Source: CAD feature listing. Evaluate the final solid. Frame: model axes, mm. Face numbers are marked on the shaded views. Round coordinates to 2 decimals unless told otherwise and drop trailing zeros. Write each loop counter-clockwise with the first axis right and the second up, starting at its lowest first coordinate (ties: lowest second). Pieces come first, ordered by that corner, then holes.
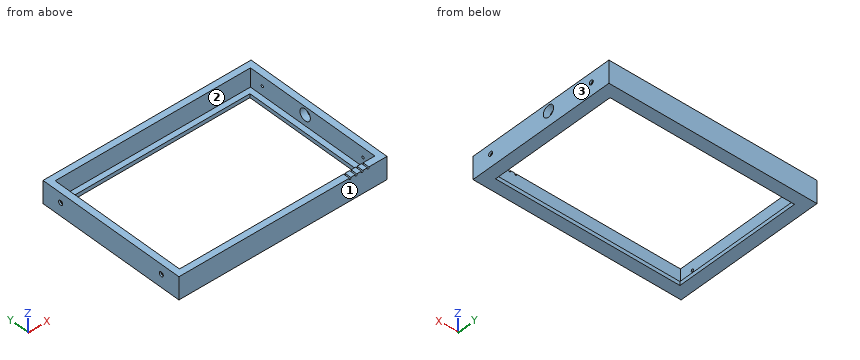
from build123d import *

# Parameters (mm, degrees)
CYLINDER027_R           = 3.5
CYLINDER027_DEPTH       = 3
CYLINDER027_PITCH_ANGLE = 90
CYLINDER026_R           = 2
CYLINDER026_DEPTH       = 9
CYLINDER026_PITCH_ANGLE = 90
ARRAY023_COUNT          = 2
ARRAY024_Y_COUNT        = 2
ARRAY024_Y_PITCH        = 174
CYLINDER011_R           = 9
CYLINDER011_DEPTH       = 12
CYLINDER011_PITCH_ANGLE = 90
CYLINDER010_R           = 1.5
CYLINDER010_DEPTH       = 11
ARRAY007_X_COUNT        = 4
ARRAY007_X_PITCH        = 9.4
ARRAY007_ROLL_ANGLE     = 90
BOX005_W                = 288
BOX005_H                = 198
BOX005_DEPTH            = 6
BOX004_W                = 325
BOX004_H                = 235
BOX004_DEPTH            = 6
BOX007_W                = 305
BOX007_H                = 215
BOX007_DEPTH            = 29
BOX006_W                = 325
BOX006_H                = 235
BOX006_DEPTH            = 29
CUT014_PLACEMENT_ANGLE  = 180


with BuildPart() as case_2_frame_cut005:
    # Cylinder027 → Cylinder027 (new body)
    with BuildSketch(Plane.XY):
        Circle(CYLINDER027_R)
    extrude(amount=CYLINDER027_DEPTH)


with BuildPart() as case_2_frame_cut005_1:
    # Cylinder027 pitch: moved
    add(case_2_frame_cut005.part.rotate(Axis((0, 0, 0), (0, 1, 0)), CYLINDER027_PITCH_ANGLE))


with BuildPart() as case_2_frame_cut005_2:
    # Cylinder027 placement: moved
    add(case_2_frame_cut005_1.part)


with BuildPart() as array024:
    # Cylinder026 → Cylinder026 (new body)
    with BuildSketch(Plane.XY):
        Circle(CYLINDER026_R)
    extrude(amount=CYLINDER026_DEPTH)


with BuildPart() as array024_1:
    # Cylinder026 pitch: moved
    add(array024.part.rotate(Axis((0, 0, 0), (0, 1, 0)), CYLINDER026_PITCH_ANGLE))


with BuildPart() as array024_2:
    # Cylinder026 placement: moved
    add(array024_1.part.moved(Location((3, 0, 0))))

    # Fusion021: union CASE_2_frame_cut005
    add(case_2_frame_cut005_2.part)


with BuildPart() as array024_3:
    # Fusion021 placement: moved
    add(array024_2.part.moved(Location((-163, 87, -14))))

    # Array023: Array024 ×2 about axis
    array023_axis = Axis((0, 87, 0), (0, 0, 1))


with BuildPart() as array024_4:
    add(array024_3.part)
    for i in range(1, ARRAY023_COUNT):
        add(array024_3.part.rotate(array023_axis, i * 360 / ARRAY023_COUNT))

    # Array024 Y: Array024 ×2


with BuildPart() as array024_5:
    add(array024_4.part)
    with Locations(*[(0, -i * ARRAY024_Y_PITCH, 0) for i in range(1, ARRAY024_Y_COUNT)]):
        add(array024_4.part)


with BuildPart() as array024_6:
    # Array024 placement: moved
    add(array024_5.part.moved(Location((0, 0, -30))))


with BuildPart() as case_2_frame_cut:
    # Cylinder011 → Cylinder011 (new body)
    with BuildSketch(Plane.XY):
        Circle(CYLINDER011_R)
    extrude(amount=CYLINDER011_DEPTH)


with BuildPart() as case_2_frame_cut_1:
    # Cylinder011 pitch: moved
    add(case_2_frame_cut.part.rotate(Axis((0, 0, 0), (0, 1, 0)), CYLINDER011_PITCH_ANGLE))


with BuildPart() as case_2_frame_cut_2:
    # Cylinder011 placement: moved
    add(case_2_frame_cut_1.part.moved(Location((151, 13, -41.5))))


with BuildPart() as obj1:
    # Cylinder010 → Cylinder010 (new body)
    with BuildSketch(Plane(origin=(-30, -25, 0), x_dir=(1, 0, 0), z_dir=(0, 0, 1))):
        Circle(CYLINDER010_R)
    extrude(amount=CYLINDER010_DEPTH)

    # Array007 X: obj1 ×4


with BuildPart() as obj1_1:
    add(obj1.part)
    with Locations(*[(i * ARRAY007_X_PITCH, 0, 0) for i in range(1, ARRAY007_X_COUNT)]):
        add(obj1.part)


with BuildPart() as obj1_2:
    # Array007 roll: moved
    add(obj1_1.part.rotate(Axis((0, 0, 0), (1, 0, 0)), ARRAY007_ROLL_ANGLE))


with BuildPart() as obj1_3:
    # Array007 placement: moved
    add(obj1_2.part.moved(Location((-103, -106.5, 55))))


with BuildPart() as obj2:
    # Box005 → Box005 (new body)
    with BuildSketch(Plane(origin=(-144, -99, 0), x_dir=(1, 0, 0), z_dir=(0, 0, 1))):
        with Locations((144, 99)):
            Rectangle(BOX005_W, BOX005_H)
    extrude(amount=BOX005_DEPTH)


with BuildPart() as case_2_frame_u001:
    # Box004 → Box004 (new body)
    with BuildSketch(Plane(origin=(-162.5, -117.5, 0), x_dir=(1, 0, 0), z_dir=(0, 0, 1))):
        with Locations((162.5, 117.5)):
            Rectangle(BOX004_W, BOX004_H)
    extrude(amount=BOX004_DEPTH)

    # Cut005: cut obj2
    add(obj2.part, mode=Mode.SUBTRACT)


with BuildPart() as case_2_frame_u001_1:
    # Cut005 placement: moved
    add(case_2_frame_u001.part.moved(Location((0, 0, 58))))


with BuildPart() as obj3:
    # Box007 → Box007 (new body)
    with BuildSketch(Plane(origin=(-152.5, -107.5, 0), x_dir=(1, 0, 0), z_dir=(0, 0, 1))):
        with Locations((152.5, 107.5)):
            Rectangle(BOX007_W, BOX007_H)
    extrude(amount=BOX007_DEPTH)


with BuildPart() as case_2_frame_back002:
    # Box006 → Box006 (new body)
    with BuildSketch(Plane(origin=(-162.5, -117.5, 0), x_dir=(1, 0, 0), z_dir=(0, 0, 1))):
        with Locations((162.5, 117.5)):
            Rectangle(BOX006_W, BOX006_H)
    extrude(amount=BOX006_DEPTH)

    # Cut006: cut obj3
    add(obj3.part, mode=Mode.SUBTRACT)


with BuildPart() as case_2_frame_back002_1:
    # Cut006 placement: moved
    add(case_2_frame_back002.part.moved(Location((0, 0, 29))))

    # Fusion018: union CASE_2_frame_u001
    add(case_2_frame_u001_1.part)

    # Cut014: cut obj1
    add(obj1_3.part, mode=Mode.SUBTRACT)


with BuildPart() as case_2_frame_back002_2:
    # Cut014 placement: moved
    add(case_2_frame_back002_1.part.rotate(Axis((0, 0, 0), (0, 1, 0)), CUT014_PLACEMENT_ANGLE))

    # Cut019: cut CASE_2_frame_cut
    add(case_2_frame_cut_2.part, mode=Mode.SUBTRACT)

    # Cut025: cut Array024
    add(array024_6.part, mode=Mode.SUBTRACT)


solid = case_2_frame_back002_2.part
1) Contact query for flat-ended pins moving along their axis: P1, Ø3.5, axis at x = 104.8, z = -30, coming from the -Y side; P2, Ø6.5, axis at y = 87, z = -44, coming from the +X side; P3, Ø5.5, axis at y = 86.5, z = -43.5, coming from the -X side. Output: stop coordinate, or through.
Taken from the geometry:
P1: stops at y = -117.5
P2: stops at x = 160
P3: stops at x = -160
2) Section query A-A on y = 13. Return the cut outline in (x, z), then the cut area to 3 significant figures.
Taken from the geometry:
outline: (-162.5, -64) - (-144, -64) - (-144, -58) - (-152.5, -58) - (-152.5, -29) - (-162.5, -29) - close; (144, -64) - (162.5, -64) - (162.5, -50.5) - (152.5, -50.5) - (152.5, -58) - (144, -58) - close; (152.5, -32.5) - (162.5, -32.5) - (162.5, -29) - (152.5, -29) - close
area: 622 mm2
3) Section query B-B on x = 42. Return the cut outline in (y, z), then the cut area to 3 significant figures.
Taken from the geometry:
outline: (-117.5, -64) - (-99, -64) - (-99, -58) - (-107.5, -58) - (-107.5, -29) - (-117.5, -29) - close; (99, -64) - (117.5, -64) - (117.5, -29) - (107.5, -29) - (107.5, -58) - (99, -58) - close
area: 802 mm2
4) Section query C-C on y = -67.5. Return the cut outline in (x, z).
Taken from the geometry:
outline: (-162.5, -64) - (-144, -64) - (-144, -58) - (-152.5, -58) - (-152.5, -29) - (-162.5, -29) - close; (144, -64) - (162.5, -64) - (162.5, -29) - (152.5, -29) - (152.5, -58) - (144, -58) - close
5) Material intervals for line 1 (Y direction, x = -161, z = -44); line 2 (X direction, y = -111.25, z = -30); line 3 (Y direction, x = -45, z = -56), sorted ascending.
Taken from the geometry:
line 1: y = -117.5 to -90.5, -83.5 to 83.5, 90.5 to 117.5
line 2: x = -162.5 to 103.3, 106.3 to 112.7, 115.7 to 122.1, 125.1 to 131.5, 134.5 to 162.5
line 3: y = -117.5 to -107.5, 107.5 to 117.5
6) Pull-direction query (Y, two-part tool) for the marked faces 1, 2 and 3; classes: released by +Y, released by -Y, zero draft, split by the parting line, or undercut.
Taken from the geometry:
face 1: released by -Y
face 2: undercut
face 3: zero draft
